from build123d import *

# Parameters (mm, degrees)
F0_R     = 17.888087
F0_R_2   = 17.8943
F1_DEPTH = 5.08


with BuildPart() as f1:
    # F0 (on Front) → F1 (new body)
    with BuildSketch(Plane.XZ):
        Polygon((56.788196, 25.584594), (-44.811804, 25.584593), (-44.811804, -27.755406), (56.788196, -27.755406), align=None)
        with Locations((-21.516809, 0)):
            Circle(F0_R, mode=Mode.SUBTRACT)
        with Locations((33.483696, 0)):
            Circle(F0_R_2, mode=Mode.SUBTRACT)
    extrude(amount=F1_DEPTH)


solid = f1.part
Model file for the job. Use its own axes, mm. Give positions to 0.01 mm unless a question says otherwise; leave off trailing zeros. Write each loop counter-clockwise with the first axis right and the second up, starting at its lowest first coordinate (ties: lowest second). Pieces come first, ordered by that corner, then holes. Notation, with made-up numbers: M 50,17.5 L 107,17.5 A7 cw 107,26.5 Z; hole C 47.25,-7.75 d10. An arc over 180 degrees is marked long. One line per item, written item: value. Start each with the question number.
Q1. Two-plate mould, pull along Z, no slides. Class faces 1 (the flat face through (5, -5.08, -1)), 2 (the cylindrical face through (-4.455, -2.504, 5.373)), 3 (the flat face through (5, -3, -27.755)): +Z half, -Z half, draft (parallel to the pull), parting line (faces both ways), or undercut.
Q2. Probe probe 1 along X at (y, z) = (-0.9, 3.5); probe 2 along X at (y, z) = (-3.3, -8); probe 3 along Z at (x, y) = (22, -1.8). List the from-to ranges inside material, lowest first. Write a range as [from, to].
Q3. Saw through at C-C, the plane x = -12.5. Write the cut outline in (y, z), plus the area to 3 significant figures.
Q4. Saw through at D-D, the plane z = 8. Write the cut outline in (x, y), plus the area to 3 significant figures.
Q5. Saw through at B-B, the plane y = -1.95. Write the cut outline in (x, z).
Q6. Saw through at A-A, the plane z = 0. Write the cut outline in (x, y).
Output values:
1. face 1: draft
1. face 2: undercut
1. face 3: -Z half
2. probe 1: x = [-44.81, -39.06], [-3.97, 15.94], [51.03, 56.79]
2. probe 2: x = [-44.81, -37.52], [-5.52, 17.48], [49.49, 56.79]
2. probe 3: z = [-27.76, -13.72], [13.72, 25.58]
3. outline: M -5.08,-27.76 L 0,-27.76 L 0,-15.45 L -5.08,-15.45 Z; M -5.08,15.45 L 0,15.45 L 0,25.58 L -5.08,25.58 Z
3. area: 114 mm²
4. outline: M -44.81,-5.08 L -37.52,-5.08 L -37.52,0 L -44.81,0 Z; M -5.52,-5.08 L 17.48,-5.08 L 17.48,0 L -5.52,0 Z; M 49.49,-5.08 L 56.79,-5.08 L 56.79,0 L 49.49,0 Z
4. area: 191 mm²
5. outline: M -44.81,-27.76 L 56.79,-27.76 L 56.79,25.58 L -44.81,25.58 Z; hole C -21.52,0 d35.78; hole C 33.48,0 d35.79
6. outline: M -44.81,-5.08 L -39.4,-5.08 L -39.4,0 L -44.81,0 Z; M -3.63,-5.08 L 15.59,-5.08 L 15.59,0 L -3.63,0 Z; M 51.38,-5.08 L 56.79,-5.08 L 56.79,0 L 51.38,0 Z
